Read the model definition and answer for the solid it produces. Units are mm, in the model's axes. Give positions to 0.01 mm unless a question says otherwise; leave off trailing zeros. Loops run counter-clockwise (first coordinate to the right, second up) from the corner with the lowest first, then second, coordinate; pieces in that order, holes last. Notation, with made-up numbers: (25, 3.25) -> (49, 3.25) arc R20 cw to (49, 9.25) -> close; hole circle Ø3 at (1.5, 68.5). An arc over 180 degrees is marked (long way). Answer as CSV lines item,"result". Start each with the question number.
```python
from build123d import *

# Parameters (mm, degrees)
F0_W     = 158
F0_H     = 210
F1_DEPTH = 0.2032
F2_R     = 19


with BuildPart() as f1:
    # F0 (on Top) → F1 (new body, symmetric)
    with BuildSketch(Plane.XY):
        with Locations((0, -85.2)):
            Rectangle(F0_W, F0_H)
        with BuildLine():
            Line((15, 0), (-15, 0))
            ThreePointArc((-15, 0), (-18.927826, 3.24357), (-16.485563, 7.713907))
            Line((-16.485563, 7.713907), (-1.485563, 13.713907))
            ThreePointArc((-1.485563, 13.713907), (0, 14), (1.485563, 13.713907))
            Line((1.485563, 13.713907), (16.485563, 7.713907))
            ThreePointArc((16.485563, 7.713907), (18.927826, 3.24357), (15, 0))
        make_face(mode=Mode.SUBTRACT)
    extrude(amount=F1_DEPTH, both=True)

    # F2
    f2_edges = [f1.edges().sort_by_distance(p)[0] for p in [
        (79, 19.8, 0),
        (-79, 19.8, 0),
        (79, -190.2, 0),
        (-79, -190.2, 0),
    ]]
    fillet(f2_edges, radius=F2_R)


solid = f1.part
```
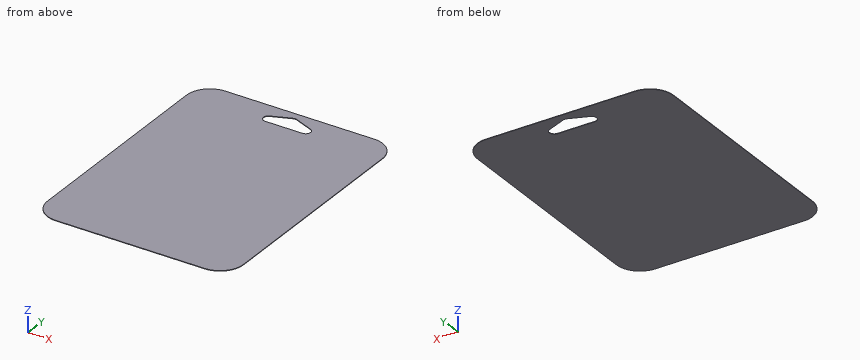
(1) Find section A-A on z = -0.05. Write down the section's boundary in (x, y), then the cut area to 3 significant figures.
(2) Find section B-B on x = -8.5. Write down the section's boundary in (y, z).
(3) Find the intervals of material crossed by line 1 along Y through (x, z) = (9, -0.1); line 2 along Y through (x, z) = (9.5, -0.1); line 3 along Y through (x, z) = (61, 0.15), in increasing order. Write a range as from..to.
(4) Find section C-C on y = 4. Write down the section's boundary in (x, z).
Answer block:
1,outline,"(-79, -171.2) arc R19 ccw to (-60, -190.2) -> (60, -190.2) arc R19 ccw to (79, -171.2) -> (79, 0.8) arc R19 ccw to (60, 19.8) -> (-60, 19.8) arc R19 ccw to (-79, 0.8) -> close; hole (-16.49, 7.71) arc R4 ccw to (-15, 0) -> (15, 0) arc R4 ccw to (16.49, 7.71) -> (1.49, 13.71) arc R4 ccw to (-1.49, 13.71) -> close"
1,area,"32,500 mm2"
2,outline,"(-190.2, -0.2) -> (0, -0.2) -> (0, 0.2) -> (-190.2, 0.2) -> close; (10.91, -0.2) -> (19.8, -0.2) -> (19.8, 0.2) -> (10.91, 0.2) -> close"
3,line 1,"y = -190.2..0, 10.71..19.8"
3,line 2,"y = -190.2..0, 10.51..19.8"
3,line 3,"y = -190.17..19.77"
4,outline,"(-78.73, -0.2) -> (-19, -0.2) -> (-19, 0.2) -> (-78.73, 0.2) -> close; (19, -0.2) -> (78.73, -0.2) -> (78.73, 0.2) -> (19, 0.2) -> close"
